Geometry check sheet. Reference: drawing and pictorial views, mm from the part's lowest x, y, z. Round coordinates to 2 decimals unless told otherwise and drop trailing zeros. Write each loop counter-clockwise with the first axis right and the second up, starting at its lowest first coordinate (ties: lowest second). Pieces come first, ordered by that corner, then holes. Notation, with made-up numbers: (66.25, -9.5) -> (92.25, -9.5) arc R27 cw to (92.25, 8.5) -> close; hole circle Ø3 at (80, -36). An arc over 180 degrees is marked (long way). Answer as a JSON object with one key per item and string values. Group by question number.
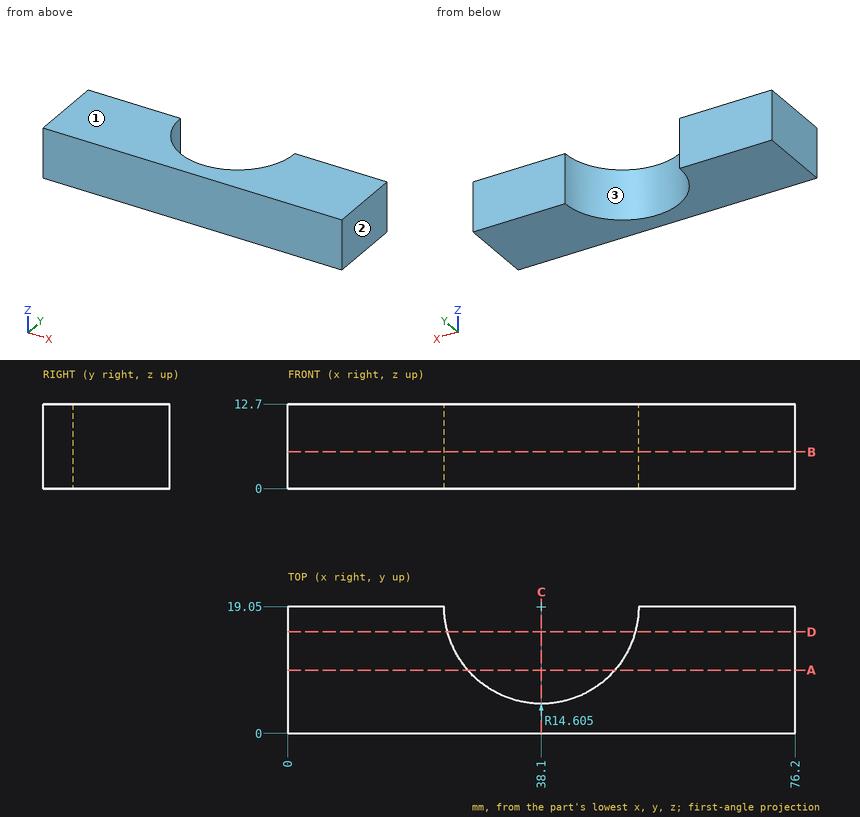
(1) Section check D-D on y = 15.25. Record the cut outline in (x, z), then the cut area to 3 significant figures.
(2) Section check C-C on x = 38.1. Record the cut outline in (y, z) (3 decimals).
(3) Scan lines: line 1 along X through (y, z) = (17.25, 3.5); line 2 along X through (y, z) = (8.25, 12); line 3 along Y through (x, z) = (45, 2). Record each from-to range of solid material in increasing order.
(4) Section check B-B on z = 5.5. Record the cut outline in (x, y) (3 decimals), then the cut area to 3 significant figures.
(5) Release check for a two-part mould opening along X. For the marked faces 1, 2 and 3 record: pulls with the +X half, pulls with the -X half, needs draft (parallel to the pull), parting line crosses it, or undercut.
(6) Section check A-A on y = 9.5. Record the cut outline in (x, z), then the cut area to 3 significant figures.
Data:
{
 "1": {"outline": "(0, 0) -> (24, 0) -> (24, 12.7) -> (0, 12.7) -> close; (52.2, 0) -> (76.2, 0) -> (76.2, 12.7) -> (52.2, 12.7) -> close", "area": "610 mm²"},
 "2": {"outline": "(0, 0) -> (4.445, 0) -> (4.445, 12.7) -> (0, 12.7) -> close"},
 "3": {"line 1": "x = 0 to 23.61, 52.59 to 76.2", "line 2": "x = 0 to 28.27, 47.93 to 76.2", "line 3": "y = 0 to 6.18"},
 "4": {"outline": "(0, 0) -> (76.2, 0) -> (76.2, 19.05) -> (52.705, 19.05) arc R14.605 cw to (23.495, 19.05) -> (0, 19.05) -> close", "area": "1,120 mm²"},
 "5": {"face 1": "needs draft", "face 2": "pulls with the +X half", "face 3": "undercut"},
 "6": {"outline": "(0, 0) -> (27.05, 0) -> (27.05, 12.7) -> (0, 12.7) -> close; (49.15, 0) -> (76.2, 0) -> (76.2, 12.7) -> (49.15, 12.7) -> close", "area": "687 mm²"}
}
